```python
from build123d import *

# Parameters (mm, degrees)
SKETCH1_W           = 195
SKETCH1_H           = 170
BOSS_EXTRUDE1_DEPTH = 6
SKETCH2_W           = 90
SKETCH2_H           = 20
CUT_EXTRUDE1_DEPTH  = 130.48841647
FILLET1_R           = 15
SKETCH3_W           = 30
SKETCH3_H           = 6
BOSS_EXTRUDE2_DEPTH = 6
CHAMFER1_SIZE       = 20
SKETCH4_R           = 1.75
CUT_EXTRUDE2_DEPTH  = 134.503745266
SKETCH7_R           = 1.75
CUT_EXTRUDE5_DEPTH  = 134.503745266
SKETCH8_R           = 1.75
CUT_EXTRUDE6_DEPTH  = 134.503745266
SKETCH6_R           = 3.5
CUT_EXTRUDE4_DEPTH  = 3
CHAMFER3_SIZE       = 6


with BuildPart() as part:
    # Sketch1 → Boss-Extrude1 (new body)
    with BuildSketch(Plane(origin=(0, 0, 0), x_dir=(1, 0, 0), z_dir=(0, 1, 0))):
        Rectangle(SKETCH1_W, SKETCH1_H)
    extrude(amount=BOSS_EXTRUDE1_DEPTH)

    # Sketch2 → Cut-Extrude1 (cut, through all)
    with BuildSketch(Plane(origin=(0, 6, 0), x_dir=(1, 0, 0), z_dir=(0, 1, 0))):
        with Locations((-22.5, -75)):
            Rectangle(SKETCH2_W, SKETCH2_H)
        with Locations((-22.5, 75)):
            Rectangle(SKETCH2_W, SKETCH2_H)
    extrude(amount=-CUT_EXTRUDE1_DEPTH, mode=Mode.SUBTRACT)

    # Fillet1
    fillet1_edges = [part.edges().sort_by_distance(p)[0] for p in [
        (-67.5, 3, 65),
        (22.5, 3, 65),
        (-67.5, 3, -65),
        (22.5, 3, -65),
    ]]
    fillet(fillet1_edges, radius=FILLET1_R)

    # Sketch3 → Boss-Extrude2 (add)
    with BuildSketch(Plane(origin=(0, 6, 0), x_dir=(1, 0, 0), z_dir=(0, 1, 0))):
        with Locations((-82.5, 88)):
            Rectangle(SKETCH3_W, SKETCH3_H)
        with Locations((-82.5, -88)):
            Rectangle(SKETCH3_W, SKETCH3_H)
    extrude(amount=-BOSS_EXTRUDE2_DEPTH)

    # Chamfer1
    chamfer1_edges = [part.edges().sort_by_distance(p)[0] for p in [
        (-97.5, 3, -91),
        (-97.5, 3, 91),
    ]]
    chamfer(chamfer1_edges, length=CHAMFER1_SIZE)

    # Sketch4 → Cut-Extrude2 (cut, through all)
    with BuildSketch(Plane(origin=(0, 6, 0), x_dir=(1, 0, 0), z_dir=(0, 1, 0))):
        with Locations(Location((-81.5, 75.766666667, 0), (0, 0, 270))):
            Circle(SKETCH4_R)
        with Locations(Location((-81.5, -75.766666667, 0), (0, 0, 90))):
            Circle(SKETCH4_R)
        with Locations(Location((-73.5, 75.766666667, 0), (0, 0, 270))):
            Circle(SKETCH4_R)
        with Locations(Location((-73.5, -75.766666667, 0), (0, 0, 90))):
            Circle(SKETCH4_R)
    extrude(amount=-CUT_EXTRUDE2_DEPTH, mode=Mode.SUBTRACT)

    # Sketch7 → Cut-Extrude5 (cut, through all)
    with BuildSketch(Plane.XZ):
        with Locations(Location((47.5, 75.05, 0), (0, 0, 270))):
            Circle(SKETCH7_R)
        with Locations(Location((72.5, 75.05, 0), (0, 0, 270))):
            Circle(SKETCH7_R)
        with Locations(Location((72.5, -75.05, 0), (0, 0, 90))):
            Circle(SKETCH7_R)
        with Locations(Location((47.5, -75.05, 0), (0, 0, 90))):
            Circle(SKETCH7_R)
    extrude(amount=-CUT_EXTRUDE5_DEPTH, mode=Mode.SUBTRACT)

    # Sketch8 → Cut-Extrude6 (cut, through all)
    with BuildSketch(Plane.XZ):
        with Locations(Location((85, 32.45, 0), (0, 0, 270))):
            Circle(SKETCH8_R)
        with Locations(Location((85, 0, 0), (0, 0, 270))):
            Circle(SKETCH8_R)
        with Locations(Location((85, -32.45, 0), (0, 0, 270))):
            Circle(SKETCH8_R)
    extrude(amount=-CUT_EXTRUDE6_DEPTH, mode=Mode.SUBTRACT)

    # Sketch6 → Cut-Extrude4 (cut)
    with BuildSketch(Plane.XZ):
        with Locations(Location((-73.5, 75.766666667, 0), (0, 0, 270))):
            Circle(SKETCH6_R)
        with Locations(Location((-81.5, 75.766666667, 0), (0, 0, 270))):
            Circle(SKETCH6_R)
        with Locations(Location((-73.5, -75.766666667, 0), (0, 0, 90))):
            Circle(SKETCH6_R)
        with Locations(Location((-81.5, -75.766666667, 0), (0, 0, 90))):
            Circle(SKETCH6_R)
        with Locations(Location((47.5, 75.05, 0), (0, 0, 270))):
            Circle(SKETCH6_R)
        with Locations(Location((72.5, 75.05, 0), (0, 0, 270))):
            Circle(SKETCH6_R)
        with Locations(Location((47.5, -75.05, 0), (0, 0, 90))):
            Circle(SKETCH6_R)
        with Locations(Location((72.5, -75.05, 0), (0, 0, 90))):
            Circle(SKETCH6_R)
        with Locations(Location((85, 32.45, 0), (0, 0, 270))):
            Circle(SKETCH6_R)
        with Locations(Location((85, 0, 0), (0, 0, 270))):
            Circle(SKETCH6_R)
        with Locations(Location((85, -32.45, 0), (0, 0, 270))):
            Circle(SKETCH6_R)
    extrude(amount=-CUT_EXTRUDE4_DEPTH, mode=Mode.SUBTRACT)

    # Chamfer3
    chamfer3_edges = [part.edges().sort_by_distance(p)[0] for p in [
        (-72.5, 0, -91),
        (-72.5, 0, 91),
    ]]
    chamfer(chamfer3_edges, length=CHAMFER3_SIZE - 0.0001)  # a hair under: the kernel refuses the full size


solid = part.part
```
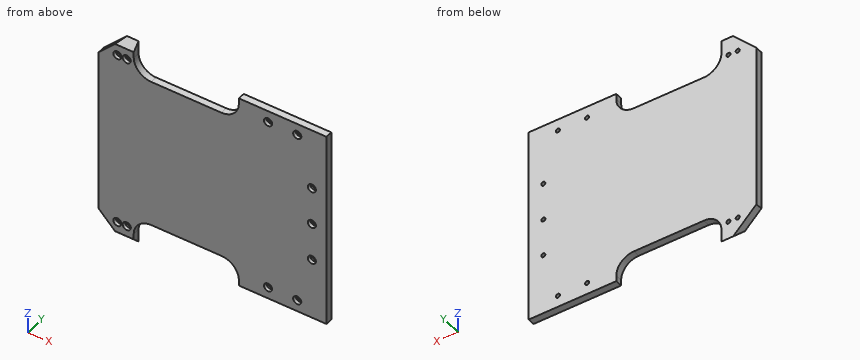
Build history of the part. All positions in model axes, mm. Round coordinates to 2 decimals unless told otherwise and drop trailing zeros. Order: outer loops, then holes, each group sorted by start corner. A loop starts at its lowest first (then second) coordinate and runs counter-clockwise, first axis right, second up. Notation, with made-up numbers: (54, 63.5) - (73, 63.5) arc R8 cw to (73, 75.5) - close; hole circle Ø2 at (-13, 86). An arc over 180 degrees is marked (long way). Use a Markdown table: item, result.
1) Flat gauge pins, fed straight in: pin 1 Ø3 at (x, z) = (47.5, -75.05) entering from +Y; pin 2 Ø5.5 at (x, z) = (47.5, 75.05) entering from -Y; pin 3 Ø2 at (x, y) = (-24, 2) entering from -Z; pin 4 Ø1.8 at (x, y) = (43.5, 1.5) entering from -Z. Where does each tip first touch, or does it go through?
Recorded:
| item | result |
|---|---|
| pin 1 | passes through |
| pin 2 | stops at y = 3 |
| pin 3 | stops at z = -65 |
| pin 4 | stops at z = -85 |
2) Wall check: L1, parallel to Z at x = 49, y = 1.25; L2, parallel to X at y = 5.35, z = 75.05. Give the ranges that are in metal, low to high.
Recorded:
| item | result |
|---|---|
| L1 | z = -85 to -78.21, -71.89 to 71.89, 78.21 to 85 |
| L2 | x = -93.45 to -83.1, -79.9 to -75.1, -71.9 to -66.66, 21.66 to 45.75, 49.25 to 70.75, 74.25 to 97.5 |
3) Saw through at B-B on x = 31. Write the cut outline in (y, z), and give its area (3 significant figures).
Recorded:
| item | result |
|---|---|
| outline | (0, -85) - (6, -85) - (6, 85) - (0, 85) - close |
| area | 1,020 mm² |
4) Saw through at A-A on y = 2. Give the number of separate pieces and of enclosed holes in the cut face, and give its area (3 significant figures).
Recorded:
| item | result |
|---|---|
| separate pieces | 1 |
| enclosed holes | 11 |
| area | 29,200 mm² |
